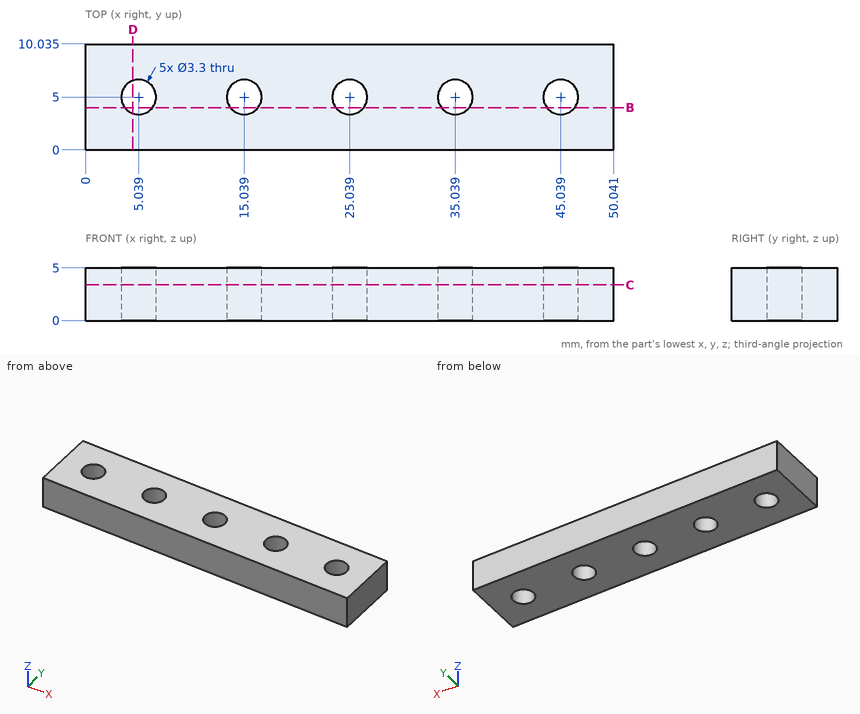
Print and shaded views of the part. All mm, measured from the part's lowest x, y and z. Coordinates: 2 decimals unless noted, no trailing zeros. Loops run counter-clockwise (first coordinate to the right, second up) from the corner with the lowest first, then second, coordinate; pieces in that order, holes last. Notation, with made-up numbers: (46, 26.25) -> (96, 26.25) arc R22 ccw to (96, 41.25) -> close; hole circle Ø9 at (15, 16.25). An arc over 180 degrees is marked (long way). Use a Markdown table: item, result. Add a question column.
Item 1: Band-saw the part on D-D on x = 4.5. Write the cut outline in (y, z) (1 decimal).
Item 2: Probe probe 1 along X at (y, z) = (5, 0.95); probe 2 along X at (y, z) = (4.25, 2.9); probe 3 along Y at (x, z) = (6, 3.2) (1 decimal). List the from-to ranges inside material, lowest first.
Item 3: Band-saw the part on C-C on z = 3.4. Give the number of separate pieces and of enclosed holes in the cut face.
Item 4: Band-saw the part on B-B on y = 4. Write the cut outline in (x, z).
Item 5: Flat gauge pin, fed straight in: P1, Ø2.5, axis at x = 35.04, y = 5, coming from the +Z side. Where does the tip first touch, or does it go through?
Geometry says:
| question | item | result |
|---|---|---|
| 1 | outline | (0, 0) -> (3.4, 0) -> (3.4, 5) -> (0, 5) -> close; (6.6, 0) -> (10, 0) -> (10, 5) -> (6.6, 5) -> close |
| 2 | probe 1 | 0 to 3.39, 6.69 to 13.39, 16.69 to 23.39, 26.69 to 33.39, 36.69 to 43.39, 46.69 to 50.04 |
| 2 | probe 2 | 0 to 3.57, 6.51 to 13.57, 16.51 to 23.57, 26.51 to 33.57, 36.51 to 43.57, 46.51 to 50.04 |
| 2 | probe 3 | 0 to 3.7, 6.3 to 10 |
| 3 | separate pieces | 1 |
| 3 | enclosed holes | 5 |
| 4 | outline | (0, 0) -> (3.73, 0) -> (3.73, 5) -> (0, 5) -> close; (6.35, 0) -> (13.73, 0) -> (13.73, 5) -> (6.35, 5) -> close; (16.35, 0) -> (23.73, 0) -> (23.73, 5) -> (16.35, 5) -> close; (26.35, 0) -> (33.73, 0) -> (33.73, 5) -> (26.35, 5) -> close; (36.35, 0) -> (43.73, 0) -> (43.73, 5) -> (36.35, 5) -> close; (46.35, 0) -> (50.04, 0) -> (50.04, 5) -> (46.35, 5) -> close |
| 5 | P1 | through |
